Work out the finished part from the listing and answer in its coordinate system (mm). Face numbers are marked on the shaded views. A direction names the side the tool comes from. Coordinates: 2 decimals unless noted, no trailing zeros. Write each loop counter-clockwise with the first axis right and the second up, starting at its lowest first coordinate (ties: lowest second). Pieces come first, ordered by that corner, then holes. Notation, with made-up numbers: (23.25, 6) - (29.25, 6) arc R14 ccw to (29.25, 33) - close; hole circle Ø9 at (-30, 50). An arc over 180 degrees is marked (long way). Use a Markdown table: item, result. Add a question column.
(1) A tool of negligible diameter and unlimited length cuts with its end or side. For the marked faces 1 and 2, from which of +Z, -Z, +X, -X, +Y, -Y can it reach the whole face along a straight path? Write none if from no direction.
(2) The part is cut by section A-A, the plane y = 0. Give the vertices of the cut face in (x, z).
(3) Given pin 1 Ø5.5 at (y, z) = (0, 12.7) entering from +X; pin 2 Ø3 at (x, y) = (9.5, 1) entering from +Z, each flat-ended and moving along its own axis, determine where each tip first touches the part or whether it passes through.
(4) The part is cut by section D-D, the plane y = 4.5. Give the vertices of the cut face in (x, z).
(5) For a pull along X with two mould halves and no side action, classify the marked faces 3, 4, 5 and 6 as released by +X, released by -X, zero draft, split by the parting line, or undercut.
(6) Find the intervals of material crossed by line 1 (Y direction, x = 2.7, z = 12.7); line 2 (Z direction, x = 4.2, y = 0); line 3 (X direction, y = 0, z = 3.75), in increasing order. Write a range as from..to.
(7) The part is cut by section C-C, the plane x = 3.75. Give the vertices of the cut face in (y, z).
(8) The part is cut by section B-B, the plane z = 12.7. Give the vertices of the cut face in (x, y), then the cut area to 3 significant figures.
from build123d import *

# Parameters (mm, degrees)
EXTRUDE1_DEPTH = 6.35
FILLET1_R      = 0.508


with BuildPart() as part:
    # Sketch1 → Extrude1 (new, symmetric)
    with BuildSketch(Plane(origin=(0, 0, 0), x_dir=(1, 0, 0), z_dir=(0, 1, 0))):
        Polygon((5.9436, -18.1864), (5.9436, -5.5626), (16.256, -5.5626), (16.256, 0), (0.381, 0), (0.381, -18.1864), align=None)
    extrude(amount=EXTRUDE1_DEPTH, both=True)

    # Sketch2 → #11 (0.191) Diameter Hole1 (revolve, cut)
    with BuildSketch(Plane(origin=(0.381, 0, 12.7), x_dir=(0, 0, 1), z_dir=(0, 1, 0))):
        Polygon((0, 0), (0, 5.5626), (2.667, 5.5626), (2.4257, 5.3213), (2.4257, 0.2413), (2.667, 0), align=None)
    revolve(axis=Axis((-5.969, 0, 12.7), (1, 0, 0)), mode=Mode.SUBTRACT)

    # Sketch4 → #10-32 Tapped Hole1 (revolve, cut)
    with BuildSketch(Plane.YZ.offset(11.1252)):
        Polygon((0, 0), (0, 5.5626), (2.667, 5.5626), (2.0193, 4.9149), (2.0193, 0.6477), (2.667, 0), align=None)
    revolve(axis=Axis((11.1252, 0, -6.35), (0, 0, 1)), mode=Mode.SUBTRACT)

    # Fillet1
    fillet1_edges = [part.edges().sort_by_distance(p)[0] for p in [
        (11.0998, 6.35, 5.5626),
        (8.3185, 6.35, 0),
        (8.3185, -6.35, 0),
        (11.0998, -6.35, 5.5626),
        (3.1623, 6.35, 18.1864),
        (3.1623, -6.35, 18.1864),
    ]]
    fillet(fillet1_edges, radius=FILLET1_R)


solid = part.part
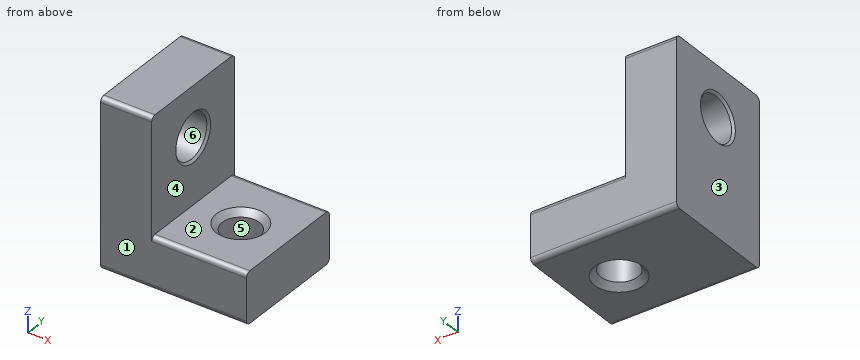
Model answer:
| question | item | result |
|---|---|---|
| 1 | face 1 | +Z, -Z, +X, -X, -Y |
| 1 | face 2 | +Z, +X, +Y, -Y |
| 2 | outline | (0.38, 0) - (8.46, 0) - (9.11, 0.65) - (9.11, 4.91) - (8.46, 5.56) - (5.94, 5.56) - (5.94, 10.03) - (5.7, 10.27) - (0.62, 10.27) - (0.38, 10.03) - close; (0.38, 15.37) - (0.62, 15.13) - (5.7, 15.13) - (5.94, 15.37) - (5.94, 18.19) - (0.38, 18.19) - close; (13.14, 0.65) - (13.79, 0) - (16.26, 0) - (16.26, 5.56) - (13.79, 5.56) - (13.14, 4.91) - close |
| 3 | pin 1 | x = 5.94 |
| 3 | pin 2 | z = 5.56 |
| 4 | outline | (0.38, 0) - (16.26, 0) - (16.26, 5.56) - (5.94, 5.56) - (5.94, 18.19) - (0.38, 18.19) - close |
| 5 | face 3 | released by -X |
| 5 | face 4 | released by +X |
| 5 | face 5 | undercut |
| 5 | face 6 | zero draft |
| 6 | line 1 | -6.35..-2.43, 2.43..6.35 |
| 6 | line 2 | 0..10.27, 15.13..18.19 |
| 6 | line 3 | 0.38..9.11, 13.14..16.26 |
| 7 | outline | (-6.35, 0.51) arc R0.51 ccw to (-5.84, 0) - (5.84, 0) arc R0.51 ccw to (6.35, 0.51) - (6.35, 17.68) arc R0.51 ccw to (5.84, 18.19) - (-5.84, 18.19) arc R0.51 ccw to (-6.35, 17.68) - close; hole circle Ø4.85 at (0, 12.7) |
| 8 | outline | (0.38, -6.35) - (5.94, -6.35) - (5.94, -2.67) - (5.7, -2.43) - (0.62, -2.43) - (0.38, -2.67) - close; (0.38, 2.67) - (0.62, 2.43) - (5.7, 2.43) - (5.94, 2.67) - (5.94, 6.35) - (0.38, 6.35) - close |
| 8 | area | 43.5 mm^2 |
